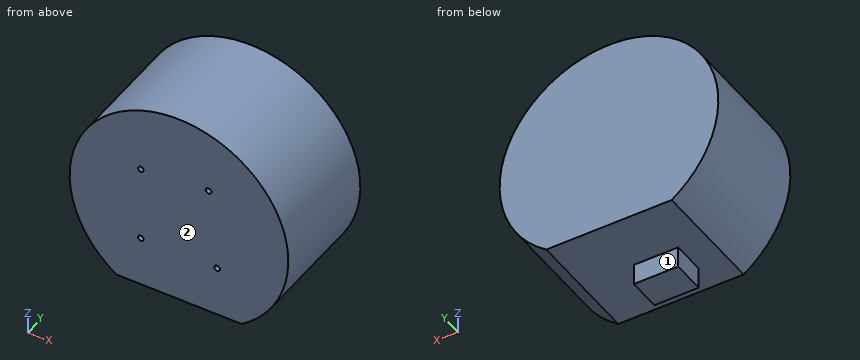
```python
from build123d import *

# Parameters (mm, degrees)
BOSS_EXTRUDE1_DEPTH = 82.55
SKETCH2_R           = 2
CUT_EXTRUDE1_DEPTH  = 5
SKETCH3_W           = 31.5
SKETCH3_H           = 23.5
BOSS_EXTRUDE2_DEPTH = 15


with BuildPart() as part:
    # Sketch1 → Boss-Extrude1 (new body)
    with BuildSketch(Plane(origin=(0, 0, 0), x_dir=(1, 0, 0), z_dir=(0, 1, 0))):
        with BuildLine():
            Line((-44.429719783, 63.5), (44.429719783, 63.5))
            ThreePointArc((44.429719783, 63.5), (0, -77.5), (-44.429719783, 63.5))
        make_face()
    extrude(amount=BOSS_EXTRUDE1_DEPTH)

    # Sketch2 → Cut-Extrude1 (cut)
    with BuildSketch(Plane.XZ):
        with Locations(Location((-27, -27.5, 0), (0, 0, 270))):
            Circle(SKETCH2_R)
        with Locations(Location((-27, 26.5, 0), (0, 0, 270))):
            Circle(SKETCH2_R)
        with Locations(Location((21, 30.5, 0), (0, 0, 270))):
            Circle(SKETCH2_R)
        with Locations(Location((27, -27.5, 0), (0, 0, 90))):
            Circle(SKETCH2_R)
    extrude(amount=-CUT_EXTRUDE1_DEPTH, mode=Mode.SUBTRACT)

    # Sketch3 → Boss-Extrude2 (add)
    with BuildSketch(Plane(origin=(0, 0, -63.5), x_dir=(-1, 0, 0), z_dir=(0, 0, -1))):
        with Locations((8.56875, 30.75)):
            Rectangle(SKETCH3_W, SKETCH3_H)
    extrude(amount=BOSS_EXTRUDE2_DEPTH)


solid = part.part
```
Build history of the part. All positions in model axes, mm. Face numbers are marked on the shaded views. A direction names the side the tool comes from. Round coordinates to 2 decimals unless told otherwise and drop trailing zeros. Write each loop counter-clockwise with the first axis right and the second up, starting at its lowest first coordinate (ties: lowest second). Pieces come first, ordered by that corner, then holes.
1) 3-axis set-ups, long thin cutter, end or side, ignore diameter. For the marked faces 1 and 2: which of +Z, -Z, +X, -X, +Y, -Y reach the whole face in a straight line?
2) Pin check, flat tips, straight feed: pin 1 (5 mm diameter, centred on y = 37.5, z = -43.5, fed in from -X); pin 2 (1.2 mm diameter, centred on x = 21.5, z = 30, fed in from -Y); pin 3 (10 mm diameter, centred on y = 47.5, z = 30.5, fed in from +X). Stop position of each tip, or through.
3) Band-saw the part on B-B, the plane z = 26.5. List the corners of the cut face in (x, y), and give its area (3 significant figures).
4) Band-saw the part on C-C, the plane y = 29. List the corners of the cut face in (x, z), and give its area (3 significant figures).
5) Band-saw the part on A-A, the plane x = 0. List the corners of the cut face in (y, z).
6) Drill centre lines: probe 1 along X at (y, z) = (1.3, -27.5); probe 2 along X at (y, z) = (43, -1); probe 3 along Z at (x, y) = (27, 1.3). Where is each one in solid material? Low to high.
7) Band-saw the part on D-D, the plane y = 76. List the corners of the cut face in (x, z).
Ans:
1. face 1: -Z, +X, -X, +Y
1. face 2: +Z, -Z, +X, -X, -Y
2. pin 1: stops at x = -65.77
2. pin 2: stops at y = 5
2. pin 3: stops at x = 73.18
3. outline: (-72.83, 0) - (-29, 0) - (-29, 5) - (-25, 5) - (-25, 0) - (72.83, 0) - (72.83, 82.55) - (-72.83, 82.55) - close
3. area: 12,000 mm2
4. outline: (-44.43, -63.5) - (-24.32, -63.5) - (-24.32, -78.5) - (7.18, -78.5) - (7.18, -63.5) - (44.43, -63.5) arc R77.5 ccw (long way) to start
4. area: 18,500 mm2
5. outline: (0, -63.5) - (19, -63.5) - (19, -78.5) - (42.5, -78.5) - (42.5, -63.5) - (82.55, -63.5) - (82.55, 77.5) - (0, 77.5) - close
6. probe 1: x = -72.46 to -29, -25 to 25, 29 to 72.46
6. probe 2: x = -77.49 to 77.49
6. probe 3: z = -63.5 to -29.5, -25.5 to 72.64
7. outline: (-44.43, -63.5) - (44.43, -63.5) arc R77.5 ccw (long way) to start
